```python
from build123d import *

# Parameters (mm, degrees)
BOSS_EXTRUDE1_DEPTH = 6
SKETCH1_3_R         = 3.6
SKETCH1_3_R_2       = 2.5
SKETCH1_3_R_3       = 2
SKETCH1_3_R_4       = 1.5
CUT_EXTRUDE1_DEPTH  = 6


with BuildPart() as part:
    # Sketch1 → Boss-Extrude1 (new body)
    with BuildSketch(Plane(origin=(0, 0, 0), x_dir=(1, 0, 0), z_dir=(0, 1, 0))):
        Polygon((-30.541760722, -55.01618123), (30.541760722, -55.01618123), (30.541760722, 55.01618123), (-30.541760722, 55.01618123), (-30.541760722, 29.2), align=None)
    extrude(amount=BOSS_EXTRUDE1_DEPTH)

    # Sketch1<3> → Cut-Extrude1 (cut)
    with BuildSketch(Plane(origin=(0, 0, 0), x_dir=(1, 0, 0), z_dir=(0, 1, 0))):
        with Locations((-20, 49.05)):
            Circle(SKETCH1_3_R)
        with Locations((20, 49.05)):
            Circle(SKETCH1_3_R)
        with Locations((-20, -49.05)):
            Circle(SKETCH1_3_R_2)
        with Locations((20, -49.05)):
            Circle(SKETCH1_3_R_2)
        with Locations((17, 12)):
            Circle(SKETCH1_3_R_3)
        with Locations((27, 12)):
            Circle(SKETCH1_3_R_3)
        with Locations((27, -18)):
            Circle(SKETCH1_3_R_3)
        with Locations((17, -18)):
            Circle(SKETCH1_3_R_3)
        with Locations((-7, -50.01618123)):
            Circle(SKETCH1_3_R_4)
        with Locations((3, -50.01618123)):
            Circle(SKETCH1_3_R_4)
        with Locations((-27, 12)):
            Circle(SKETCH1_3_R_3)
        with Locations((-17, 12)):
            Circle(SKETCH1_3_R_3)
        with Locations((6, -40)):
            Circle(SKETCH1_3_R_4)
        with Locations((16, -40)):
            Circle(SKETCH1_3_R_4)
    extrude(amount=CUT_EXTRUDE1_DEPTH, mode=Mode.SUBTRACT)


solid = part.part
```
For this review, take the finished solid that the model builds, in its own axes (mm). Round coordinates to 2 decimals unless told otherwise and drop trailing zeros. Write each loop counter-clockwise with the first axis right and the second up, starting at its lowest first coordinate (ties: lowest second). Pieces come first, ordered by that corner, then holes. Notation, with made-up numbers: (-31.75, -27) -> (-19.75, -27) arc R21 ccw to (-19.75, -19) -> close; hole circle Ø10 at (77.5, 28). An arc over 180 degrees is marked (long way). One line per question, with ' | ' between items. Start each with the question number.
1) Add section D-D (x = 6). Write out the cut boundary in (y, z).
2) Mouldability with a two-part tool opening along Z and no side actions: class faces 1 (the flat face through (0, 0, -1)), 2 (the flat face through (0, 3, -55.016)), 3 (the cylindrical face through (-21.84, 2.96, 47.36)) as +Z half, -Z half, draft (parallel to the pull), parting line (faces both ways), or undercut.
3) Add section B-B (x = 27). Write out the cut boundary in (y, z), and give its area (3 significant figures).
4) Wall thickness on line 1 along X through (y, z) = (2.5, -12); line 2 along Z through (x, y) = (20, 3.95); line 3 along X through (y, z) = (3.4, -49.05): over which ranges is each line inside the solid? List them lowest first.
5) Add section A-A (z = 18). Write out the cut boundary in (x, y).
6) Add section C-C (z = -12). Write out the cut boundary in (x, y).
Reported:
1) outline: (0, -55.02) -> (6, -55.02) -> (6, 38.5) -> (0, 38.5) -> close; (0, 41.5) -> (6, 41.5) -> (6, 55.02) -> (0, 55.02) -> close
2) face 1: draft | face 2: -Z half | face 3: undercut
3) outline: (0, -55.02) -> (6, -55.02) -> (6, -14) -> (0, -14) -> close; (0, -10) -> (6, -10) -> (6, 16) -> (0, 16) -> close; (0, 20) -> (6, 20) -> (6, 55.02) -> (0, 55.02) -> close | area: 612 mm²
4) line 1: x = -30.54 to -29, -25 to -19, -15 to 15, 19 to 25, 29 to 30.54 | line 2: z = -55.02 to -52.65, -45.45 to 46.55, 51.55 to 55.02 | line 3: x = -30.54 to -23.6, -16.4 to 16.4, 23.6 to 30.54
5) outline: (-30.54, 0) -> (15, 0) -> (15, 6) -> (-30.54, 6) -> close; (19, 0) -> (25, 0) -> (25, 6) -> (19, 6) -> close; (29, 0) -> (30.54, 0) -> (30.54, 6) -> (29, 6) -> close
6) outline: (-30.54, 0) -> (-29, 0) -> (-29, 6) -> (-30.54, 6) -> close; (-25, 0) -> (-19, 0) -> (-19, 6) -> (-25, 6) -> close; (-15, 0) -> (15, 0) -> (15, 6) -> (-15, 6) -> close; (19, 0) -> (25, 0) -> (25, 6) -> (19, 6) -> close; (29, 0) -> (30.54, 0) -> (30.54, 6) -> (29, 6) -> close
